Input: part model. Units: mm. Frame: model coordinates. Coordinates: 2 decimals unless noted, no trailing zeros. Loops run counter-clockwise (first coordinate to the right, second up) from the corner with the lowest first, then second, coordinate; pieces in that order, holes last.
```python
from build123d import *

# Parameters (mm, degrees)
BOSS_EXTRUDE1_DEPTH         = 158.750001
BOSS_EXTRUDE1_DEPTH_BACK    = 158.750001
SKETCH3_W                   = 50.8
SKETCH3_H                   = 25.4
SKETCH3_W_2                 = 47.625
SKETCH3_H_2                 = 22.225
SKETCH4_R                   = 14.2875
CUT_EXTRUDE1_DEPTH          = 39.37
F_10_CLEARANCE_HOLE1_D      = 4.9784
F_10_CLEARANCE_HOLE2_D      = 4.9784
F_10_CLEARANCE_HOLE3_D      = 4.9784
F_20_0_161_DIAMETER_HOLE1_D = 4.0894
F_10_CLEARANCE_HOLE4_D      = 4.9784
F_10_CLEARANCE_HOLE4_DEPTH  = 12.7
F_10_CLEARANCE_HOLE4_TIP    = 1.495662253


with BuildPart() as part:
    # Sketch3 → Boss-Extrude1 (new, two sides: drawn at the far end of the back side and taken through both)
    with BuildSketch(Plane.XY.offset(-BOSS_EXTRUDE1_DEPTH_BACK)):
        Rectangle(SKETCH3_W, SKETCH3_H)
        Rectangle(SKETCH3_W_2, SKETCH3_H_2, mode=Mode.SUBTRACT)
    extrude(amount=BOSS_EXTRUDE1_DEPTH + BOSS_EXTRUDE1_DEPTH_BACK)

    # Sketch4 → Cut-Extrude1 (cut)
    with BuildSketch(Plane(origin=(0, 12.7, 0), x_dir=(1, 0, 0), z_dir=(0, 1, 0))):
        with Locations(Location((9.525, 95.250000508, 0), (0, 0, 180))):
            Circle(SKETCH4_R)
        with Locations(Location((0, -21.863697987, 0), (0, 0, 180))):
            Circle(SKETCH4_R)
    extrude(amount=-CUT_EXTRUDE1_DEPTH, mode=Mode.SUBTRACT)

    # #10 Clearance Hole1 (through all)
    with Locations(Plane(origin=(0, 12.7, 0), x_dir=(1, 0, 0), z_dir=(0, 1, 0))):
        with Locations((-17.960512242, -3.903185745), (17.960512242, -39.824210229)):
            Hole(F_10_CLEARANCE_HOLE1_D / 2)

    # #10 Clearance Hole2 (through all)
    with Locations(Plane.ZY.offset(25.4)):
        with Locations((50.549668409, 2.425), (75.949668409, 2.425)):
            Hole(F_10_CLEARANCE_HOLE2_D / 2)

    # #10 Clearance Hole3 (through all)
    with Locations(Plane(origin=(0, 12.7, 0), x_dir=(1, 0, 0), z_dir=(0, 1, 0))):
        with Locations((-19.05, -51.113080493), (-19.05, -89.213080493), (19.05, -89.213080493), (19.05, -152.400000508), (-19.05, -152.400000508)):
            Hole(F_10_CLEARANCE_HOLE3_D / 2)

    # #20 (0.161) Diameter Hole1 (through all)
    with Locations(Plane(origin=(0, -12.7, 0), x_dir=(-1, 0, 0), z_dir=(0, -1, 0))):
        with Locations((-5.525370258, 77.925700755), (-13.524629742, 112.57430026)):
            Hole(F_20_0_161_DIAMETER_HOLE1_D / 2)

    # #10 Clearance Hole4
    with Locations(Plane(origin=(25.4, 0, 0), x_dir=(0, 0, -1), z_dir=(1, 0, 0))):
        with Locations((146.050000508, 0), (-105.917999492, 0)):
            Hole(F_10_CLEARANCE_HOLE4_D / 2, depth=F_10_CLEARANCE_HOLE4_DEPTH)
            with Locations((0, 0, -(F_10_CLEARANCE_HOLE4_DEPTH + F_10_CLEARANCE_HOLE4_TIP / 2))):  # 118° drill point
                Cone(0, F_10_CLEARANCE_HOLE4_D / 2, F_10_CLEARANCE_HOLE4_TIP, mode=Mode.SUBTRACT)


solid = part.part
```
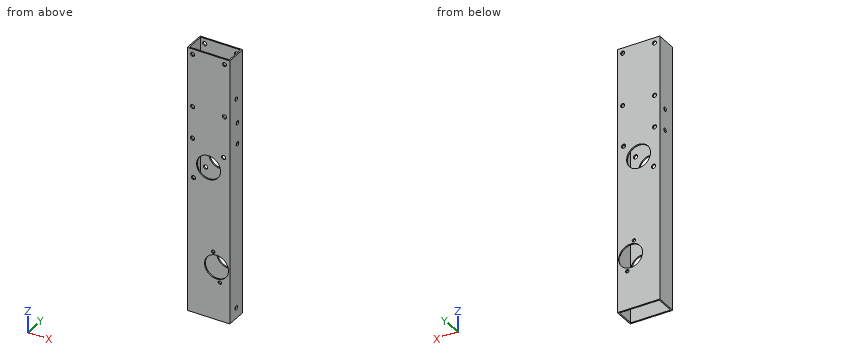
Item 1: Line query: L1, parallel to X at y = 5, z = 101; L2, parallel to Y at x = 5, z = 71; L3, parallel to Z at x = -19.05, y = 12.05. Output: solid intervals per line, ascending.
Result:
L1: x = -25.4 to -23.81, 23.81 to 25.4
L2: y = -12.7 to -11.11, 11.11 to 12.7
L3: z = -158.75 to 1.67, 6.14 to 48.62, 53.6 to 86.72, 91.7 to 149.91, 154.89 to 158.75
Item 2: Section query B-B (x = -8.5). Output: boundary loops of the cut face in (y, z), then the cut area to 3 significant figures.
Result:
outline: (-12.7, -158.75) - (-11.11, -158.75) - (-11.11, 10.38) - (-12.7, 10.38) - close; (-12.7, 33.35) - (-11.11, 33.35) - (-11.11, 158.75) - (-12.7, 158.75) - close; (11.11, -158.75) - (12.7, -158.75) - (12.7, 10.38) - (11.11, 10.38) - close; (11.11, 33.35) - (12.7, 33.35) - (12.7, 158.75) - (11.11, 158.75) - close
area: 935 mm2
Item 3: Contact query for a flat-ended pin moving along its axis: P1, Ø3, axis at x = 19.05, z = 152.4, coming from the -Y side. Output: stop coordinate, or through.
Result:
P1: passes through
Item 4: Section query A-A (z = -57.5). Output: boundary loops of the cut face in (x, y), then the cut area to 3 significant figures.
Result:
outline: (-25.4, -12.7) - (25.4, -12.7) - (25.4, 12.7) - (-25.4, 12.7) - close; hole (-23.81, -11.11) - (23.81, -11.11) - (23.81, 11.11) - (-23.81, 11.11) - close
area: 232 mm2
